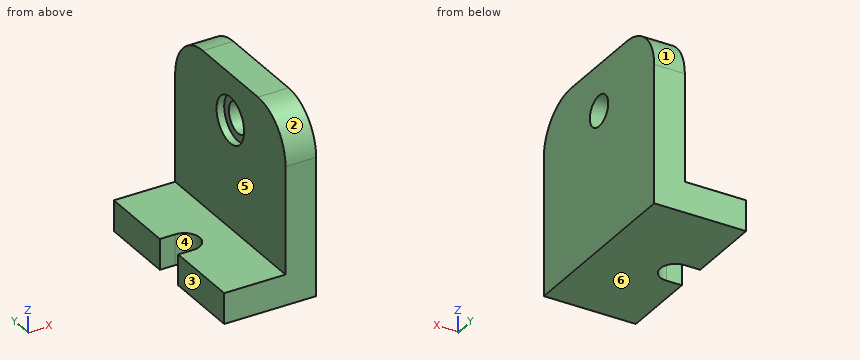
from build123d import *

# Parameters (mm, degrees)
F1_DEPTH = 76.2
F2_R     = 12.7
F3_DEPTH = 76.201
F4_W     = 12.7
F4_H     = 25.4
F5_DEPTH = 25.401
F7_R     = 38.1
F6_R     = 19.05
F8_DEPTH = 6.35


with BuildPart() as f1:
    # F0 (on Front) → F1 (new body, symmetric)
    with BuildSketch(Plane.XZ):
        Polygon((-76.2, 0), (0, 0), (0, 152.4), (-25.4, 152.4), (-25.4, 25.4), (-76.2, 25.4), align=None)
    extrude(amount=F1_DEPTH, both=True)

    # F2 (on Right) → F3 (cut, through all)
    with BuildSketch(Plane.YZ):
        with Locations((0, 114.3)):
            Circle(F2_R)
    extrude(amount=-F3_DEPTH, mode=Mode.SUBTRACT)

    # F4 (on face) → F5 (cut, through all)
    with BuildSketch(Plane.XY.offset(25.4)):
        with Locations((-69.85, 0)):
            Rectangle(F4_W, F4_H)
        with BuildLine():
            ThreePointArc((-63.5, -12.7), (-50.8, 0), (-63.5, 12.7))
            Line((-63.5, 12.7), (-63.5, -12.7))
        make_face()
    extrude(amount=-F5_DEPTH, mode=Mode.SUBTRACT)

    # F7
    f7_edges = [f1.edges().sort_by_distance(p)[0] for p in [
        (-12.7, 76.2, 152.4),
        (-12.7, -76.2, 152.4),
    ]]
    fillet(f7_edges, radius=F7_R)

    # F6 (on face) → F8 (cut)
    with BuildSketch(Plane(origin=(-25.4, 0, 0), x_dir=(0, -1, 0), z_dir=(-1, 0, 0))):
        with Locations((0, 114.3)):
            Circle(F6_R)
    extrude(amount=-F8_DEPTH, mode=Mode.SUBTRACT)


solid = f1.part
Check sheet for the modelled part. Datum: model origin and axes. Units: mm. Face numbers are marked on the shaded views. A direction names the side the tool comes from. Coordinates: 2 decimals unless noted, no trailing zeros. Loops run counter-clockwise (first coordinate to the right, second up) from the corner with the lowest first, then second, coordinate; pieces in that order, holes last. Notation, with made-up numbers: (41, 2.5) -> (88, 2.5) arc R9 ccw to (88, 16.5) -> close; hole circle Ø4 at (-16.5, 42.25). An arc over 180 degrees is marked (long way). Answer in a Markdown table with one row per item.
1. Access from +Z, -Z, +X, -X, +Y, -Y to the whole of each face (thin tool, end or side, straight path). Record for the marked faces 5 and 6.
Check values:
| item | result |
|---|---|
| face 5 | +Z, -X, +Y, -Y |
| face 6 | -Z, +X, -X, +Y, -Y |
2. Material ranges on line 1 along Z through (x, y) = (-10.75, 0); line 2 along Y through (x, z) = (-20, 114); line 3 along Y through (x, z) = (-11, 114), recorded low to high. Write a range as [from, to].
Check values:
| item | result |
|---|---|
| line 1 | z = [0, 101.6], [127, 152.4] |
| line 2 | y = [-76.2, -19.05], [19.05, 76.2] |
| line 3 | y = [-76.2, -12.7], [12.7, 76.2] |
3. Release check for a two-part mould opening along Y. For the marked faces 1, 2, 3 and 4 record: released by +Y, released by -Y, zero draft, split by the parting line, or undercut.
Check values:
| item | result |
|---|---|
| face 1 | released by +Y |
| face 2 | released by -Y |
| face 3 | zero draft |
| face 4 | undercut |
4. Go/stop test with flat-tipped pins: pin 1 (15 mm diameter, centred on x = -61.5, y = -5.5, fed in from +Z); pin 2 (6 mm diameter, centred on y = 13.5, z = 135, fed in from -X). Record where each tip stops, or that it passes through.
Check values:
| item | result |
|---|---|
| pin 1 | stops at z = 25.4 |
| pin 2 | stops at x = -25.4 |
5. Sectioned sample at A-A, the plane y = 0. Record the boundary of the cut face in (x, z).
Check values:
| item | result |
|---|---|
| outline | (-50.8, 0) -> (0, 0) -> (0, 101.6) -> (-19.05, 101.6) -> (-19.05, 95.25) -> (-25.4, 95.25) -> (-25.4, 25.4) -> (-50.8, 25.4) -> close; (-25.4, 133.35) -> (-19.05, 133.35) -> (-19.05, 127) -> (0, 127) -> (0, 152.4) -> (-25.4, 152.4) -> close |
6. Sectioned sample at B-B, the plane x = -55. Record the boundary of the cut face in (y, z), then the cut area to 3 significant figures.
Check values:
| item | result |
|---|---|
| outline | (-76.2, 0) -> (-9.44, 0) -> (-9.44, 25.4) -> (-76.2, 25.4) -> close; (9.44, 0) -> (76.2, 0) -> (76.2, 25.4) -> (9.44, 25.4) -> close |
| area | 3,390 mm2 |
7. Sectioned sample at D-D, the plane x = -35. Record the boundary of the cut face in (y, z), then the cut area to 3 significant figures.
Check values:
| item | result |
|---|---|
| outline | (-76.2, 0) -> (76.2, 0) -> (76.2, 25.4) -> (-76.2, 25.4) -> close |
| area | 3,870 mm2 |
8. Sectioned sample at C-C, the plane z = 20.5. Record the boundary of the cut face in (x, y), then the cut area to 3 significant figures.
Check values:
| item | result |
|---|---|
| outline | (-76.2, -76.2) -> (0, -76.2) -> (0, 76.2) -> (-76.2, 76.2) -> (-76.2, 12.7) -> (-63.5, 12.7) arc R12.7 cw to (-63.5, -12.7) -> (-76.2, -12.7) -> close |
| area | 11,000 mm2 |
